Verification items for the finished model (mm, model axes). Face numbers are marked on the shaded views. A direction names the side the tool comes from. Coordinates: 2 decimals unless noted, no trailing zeros. Order: outer loops, then holes, each group sorted by start corner. A loop starts at its lowest first (then second) coordinate and runs counter-clockwise, first axis right, second up. Notation, with made-up numbers: M 37,32 L 74,32 A32 ccw 74,61 Z; hole C 6,44.5 d9. An arc over 180 degrees is marked long. Return JSON: item names as keys, results as strings.
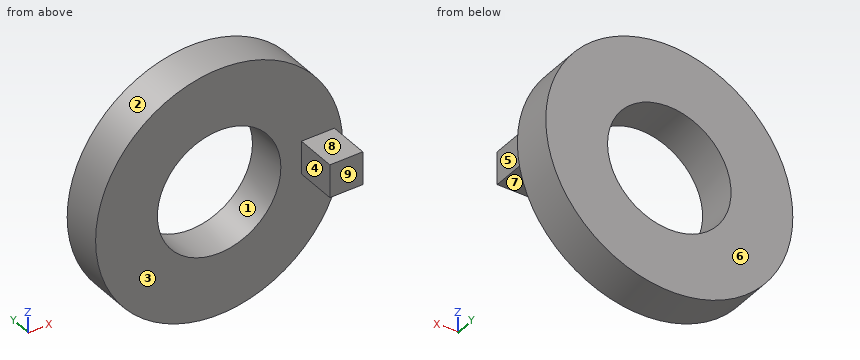
```python
from build123d import *

# Parameters (mm, degrees)
F0_R     = 75
F1_DEPTH = 25
F2_R     = 37.5
F3_DEPTH = 25
F4_W     = 20
F4_H     = 20
F5_DEPTH = 25


with BuildPart() as f1:
    # F0 (on Front) → F1 (new body)
    with BuildSketch(Plane.XZ):
        Circle(F0_R)
    extrude(amount=F1_DEPTH)

    # F2 (on face) → F3 (cut)
    with BuildSketch(Plane.XZ.offset(25)):
        Circle(F2_R)
    extrude(amount=-F3_DEPTH, mode=Mode.SUBTRACT)

    # F4 (on face) → F5 (join)
    with BuildSketch(Plane.XZ.offset(25)):
        with Locations((60, 0.96703)):
            Rectangle(F4_W, F4_H)
    extrude(amount=F5_DEPTH)


solid = f1.part
```
Q1. Material ranges on line 1 along Z through (x, y) = (0, -17); line 2 along Y through (x, z) = (9, -54.5); line 3 along Z through (x, y) = (60, -46.5), recorded low to high.
Values:
{"line 1": "-75 to -37.5, 37.5 to 75", "line 2": "-25 to 0", "line 3": "-9.03 to 10.97"}
Q2. Cross-section at A-A, the plane x = 0. Record the boundary of the cut face in (y, z).
Values:
{"outline": "M -25,-75 L 0,-75 L 0,-37.5 L -25,-37.5 Z; M -25,37.5 L 0,37.5 L 0,75 L -25,75 Z"}
Q3. Cross-section at B-B, the plane z = 0. Record the boundary of the cut face in (x, y), and give its area (4 significant figures).
Values:
{"outline": "M -75,-25 L -37.5,-25 L -37.5,0 L -75,0 Z; M 37.5,-25 L 50,-25 L 50,-50 L 70,-50 L 70,-25 L 75,-25 L 75,0 L 37.5,0 Z", "area": "2,375 mm^2"}
Q4. Draft check along X on the marked faces 1, 2, 3 and 4. Enter one of: pulls with the +X half, pulls with the -X half, needs draft (parallel to the pull), parting line crosses it, or undercut.
Values:
{"face 1": "undercut", "face 2": "parting line crosses it", "face 3": "needs draft", "face 4": "pulls with the -X half"}
Q5. Cross-section at C-C, the plane y = -17.5. Record the boundary of the cut face in (x, z), and give its area (3 significant figures).
Values:
{"outline": "C 0,0 d150; hole C 0,0 d75", "area": "13,300 mm^2"}
Q6. Cross-section at D-D, the plane z = -17.5. Record the boundary of the cut face in (x, y), and give its area (3 significant figures).
Values:
{"outline": "M -72.93,-25 L -33.17,-25 L -33.17,0 L -72.93,0 Z; M 33.17,-25 L 72.93,-25 L 72.93,0 L 33.17,0 Z", "area": "1,990 mm^2"}
Q7. Go/stop test with flat-tipped pins: pin 1 (8 mm diameter, centred on x = -40.5, y = -12, fed in from -Z); pin 2 (6 mm diameter, centred on y = -17, z = -48.5, fed in from -X); pin 3 (16 mm diameter, centred on y = -42.5, z = 5, fed in from +X). Record where each tip stops, or that it passes through.
Values:
{"pin 1": "z = -65.52", "pin 2": "x = -59.62", "pin 3": "x = 70"}
Q8. Tool access check on the marked faces 5, 6, 7, 8 and 9. Record the directions out of +Z, -Z, +X, -X, +Y, -Y that give a thin tool (end or side, any length) a straight path to the whole face; none if there is none.
Values:
{"face 5": "+Z, -Z, +X, -Y", "face 6": "+Z, -Z, +X, -X, +Y", "face 7": "-Z, +X, -X, -Y", "face 8": "+Z, +X, -X, -Y", "face 9": "+Z, -Z, +X, -X, -Y"}
